CAD build for the part. Positions are in the model's coordinates, mm. A direction names the side the tool comes from. Round coordinates to 2 decimals unless told otherwise and drop trailing zeros. Order: outer loops, then holes, each group sorted by start corner. A loop starts at its lowest first (then second) coordinate and runs counter-clockwise, first axis right, second up. Notation, with made-up numbers: M 19,-15 L 72,-15 A12 ccw 72,-1 Z; hole C 87,38 d10. An arc over 180 degrees is marked long. Answer as a JSON object with one key per item and string values.
```python
from build123d import *

# Parameters (mm, degrees)
BOSS_EXTRUDE1_DEPTH   = 2
SKETCH2_R             = 2
CUT_EXTRUDE1_DEPTH    = 2
SKETCH3_R             = 5
CUT_EXTRUDE2_DEPTH    = 2
F_3_0MM_DOWEL_HOLE2_D = 3


with BuildPart() as part:
    # Sketch1 → Boss-Extrude1 (new body)
    with BuildSketch(Plane.XY):
        with BuildLine():
            Line((0, 7), (33, 7))
            ThreePointArc((33, 7), (44.66919932, 8.739971416), (55.323194976, 13.808510638))
            ThreePointArc((55.323194976, 13.808510638), (57.187644216, 14.695505002), (59.229754097, 15))
            Line((59.229754097, 15), (68, 15))
            ThreePointArc((68, 15), (72.949747468, 12.949747468), (75, 8))
            Line((75, 8), (75, 0))
            ThreePointArc((75, 0), (72.949747468, -4.949747468), (68, -7))
            Line((68, -7), (0, -7))
            ThreePointArc((0, -7), (-7, 0), (0, 7))
        make_face()
    extrude(amount=BOSS_EXTRUDE1_DEPTH)

    # Sketch2 → Cut-Extrude1 (cut)
    with BuildSketch(Plane.XY.offset(2)):
        Circle(SKETCH2_R)
        with Locations((8, 0)):
            Circle(SKETCH2_R)
        with Locations((16, 0)):
            Circle(SKETCH2_R)
    extrude(amount=-CUT_EXTRUDE1_DEPTH, mode=Mode.SUBTRACT)

    # Sketch3 → Cut-Extrude2 (cut)
    with BuildSketch(Plane.XY.offset(2)):
        with Locations((64, 4)):
            Circle(SKETCH3_R)
    extrude(amount=-CUT_EXTRUDE2_DEPTH, mode=Mode.SUBTRACT)

    # Ø3.0mm Dowel Hole2 (through all)
    with Locations(Plane.XY.offset(2)):
        with Locations((29, -3), (37, -3), (37, 3)):
            Hole(F_3_0MM_DOWEL_HOLE2_D / 2)


solid = part.part
```
Item 1: Saw through at A-A on x = 64. List the corners of the cut face in (y, z), and give its area (3 significant figures).
Worked answers:
{"outline": "M -7,0 L -1,0 L -1,2 L -7,2 Z; M 9,0 L 15,0 L 15,2 L 9,2 Z", "area": "24.0 mm2"}
Item 2: Saw through at C-C on y = 5.5. List the corners of the cut face in (x, z), and give its area (3 significant figures).
Worked answers:
{"outline": "M -4.33,0 L 59.23,0 L 59.23,2 L -4.33,2 Z; M 68.77,0 L 75,0 L 75,2 L 68.77,2 Z", "area": "140 mm2"}
Item 3: Drop flat-ended pins along their axis: pin 1 Ø1.8 at (x, y) = (37, 3) entering from -Z; pin 2 Ø0.6 at (x, z) = (19, 0.5) entering from +Y. Give the stop position or say it passes through.
Worked answers:
{"pin 1": "passes through", "pin 2": "stops at y = 7"}
Item 4: Saw through at B-B on z = 0.3. List the corners of the cut face in (x, y).
Worked answers:
{"outline": "M 0,-7 L 68,-7 A7 ccw 75,0 L 75,8 A7 ccw 68,15 L 59.23,15 A7 ccw 55.32,13.81 A40 cw 33,7 L 0,7 A7 ccw Z; hole C 0,0 d4; hole C 8,0 d4; hole C 16,0 d4; hole C 29,-3 d3; hole C 37,-3 d3; hole C 37,3 d3; hole C 64,4 d10"}
Item 5: Wall check: line 1 along Y through (x, z) = (64, 0.4); line 2 along Y through (x, z) = (16, 0.95); line 3 along Y through (x, z) = (37, 1.05). Give the ranges that are in metal, low to high. Write a range as [from, to].
Worked answers:
{"line 1": "y = [-7, -1], [9, 15]", "line 2": "y = [-7, -2], [2, 7]", "line 3": "y = [-7, -4.5], [-1.5, 1.5], [4.5, 7.2]"}
Item 6: Saw through at D-D on x = 37. List the corners of the cut face in (y, z).
Worked answers:
{"outline": "M -7,0 L -4.5,0 L -4.5,2 L -7,2 Z; M -1.5,0 L 1.5,0 L 1.5,2 L -1.5,2 Z; M 4.5,0 L 7.2,0 L 7.2,2 L 4.5,2 Z"}
Item 7: 3-axis set-ups, long thin cutter, end or side, ignore diameter. For faces 1 (the cylindrical face through (73, -4.9, 1)), 2 (the flat face through (16, 7, 1)): which of +Z, -Z, +X, -X, +Y, -Y reach the whole face in a straight line?
Worked answers:
{"face 1": "+Z, -Z, +X, -Y", "face 2": "+Z, -Z, -X, +Y"}
